Answer from the drawing. Dimensions are ordinates in mm from the lowest x, y and z of the part. A direction names the side the tool comes from. Give positions to 0.01 mm unless a question says otherwise; leave off trailing zeros. Write each loop counter-clockwise with the first axis right and the second up, starting at its lowest first coordinate (ties: lowest second). Pieces come first, ordered by that corner, then holes. Notation, with made-up numbers: M -1.5,18 L 20.5,18 A8 ccw 20.5,28 Z; hole C 9,4 d8. An arc over 180 degrees is marked long. Write each question's results on one line, items separated by ' | '. Start each with the question number.
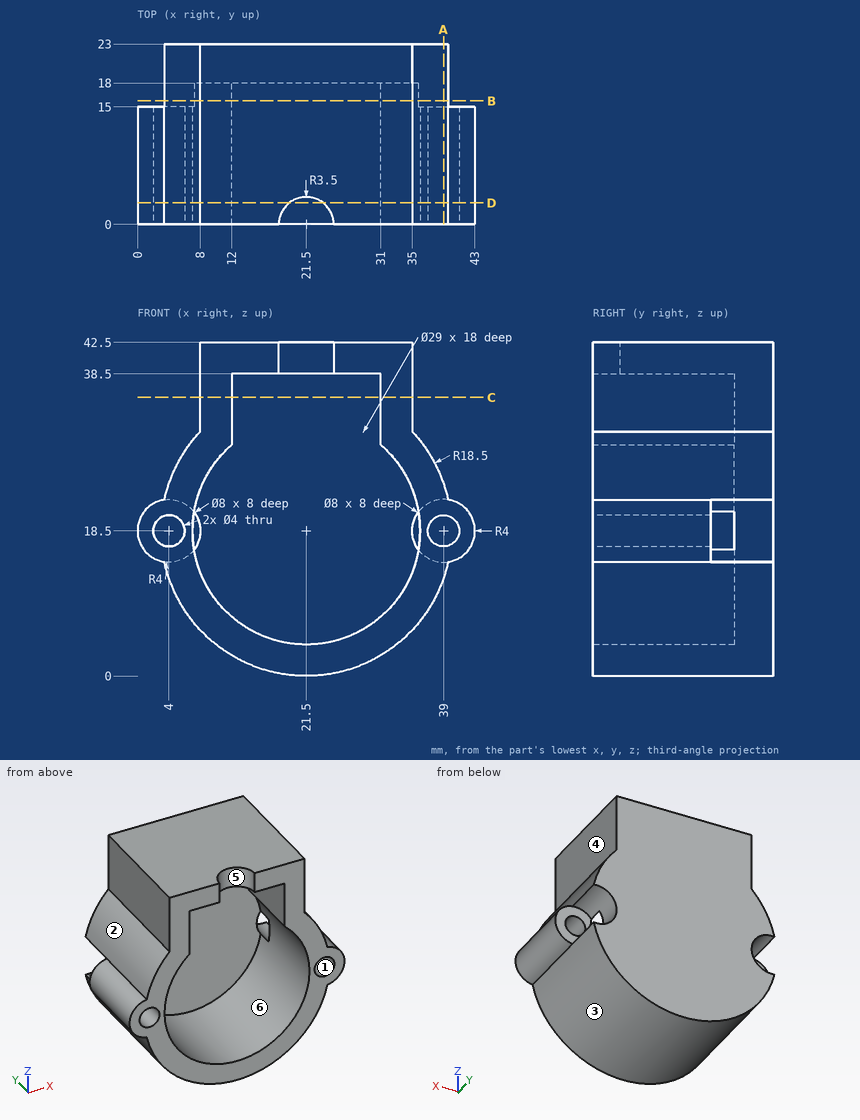
Item 1: Straight lines are drawn through the part: line 1 (X direction, y = 7.25, z = 18); line 2 (X direction, y = 16.25, z = 33); line 3 (Y direction, x = 27.5, z = 27.5). For each, find the intervals that lie inside material, in ascending order.
Item 2: For the marked faces 4, 5 and 6, determine the directions among +Z, -Z, +X, -X, +Y, -Y from which every point of the face is accessible in a straight line to the end or side of a thin tool.
Item 3: Section B-B, the plane y = 15.75 is taken. Determine the outline of the cut face in (x, z), then the cut area to 3 significant figures.
Item 4: Given P1, Ø3.5, axis at x = 3.5, z = 18.5, coming from the +Y side; P2, Ø5.5, axis at y = 9, z = 37.5, coming from the -X side; P3, Ø1.5, axis at y = 3, z = 27.5, coming from the +X side; P4, Ø3.5, axis at x = 4, z = 18.5, coming from the +Y side, each flat-ended and moving along its own axis, determine where each tip first touches the part or whether it passes through.
Item 5: Section C-C, the plane z = 35.5 is taken. Determine the outline of the cut face in (x, y).
Item 6: Determine the mould class of the marked faces 1, 2 and 3 for opening direction Z: +Z half, -Z half, draft (parallel to the pull), parting line (faces both ways), or undercut.
Item 7: Section A-A, the plane x = 39 is taken. Determine the outline of the cut face in (y, z).
Item 8: Section D-D, the plane y = 2.75 is taken. Determine the outline of the cut face in (x, z) (1 decimal).
Worked out:
1) line 1: x = 0.03 to 2.06, 5.94 to 7.01, 35.99 to 37.06, 40.94 to 42.97 | line 2: x = 8 to 12, 31 to 35 | line 3: y = 18 to 23
2) face 4: +Z, +X, +Y, -Y | face 5: +Z, -Y | face 6: -Y
3) outline: M 3.43,14.54 A18.5 ccw 39.57,14.54 A4 cw 35.8,16.1 A14.5 cw 7.2,16.1 A4 cw Z; M 3.43,22.46 A4 cw 7.2,20.9 A14.5 cw 12,29.45 L 12,38.5 L 31,38.5 L 31,29.45 A14.5 cw 35.8,20.9 A4 cw 39.57,22.46 A18.5 ccw 35,31.15 L 35,42.5 L 8,42.5 L 8,31.15 A18.5 ccw Z | area: 429 mm²
4) P1: stops at y = 15 | P2: stops at x = 8 | P3: stops at x = 38.06 | P4: passes through
5) outline: M 8,0 L 12,0 L 12,18 L 31,18 L 31,0 L 35,0 L 35,23 L 8,23 Z
6) face 1: undercut | face 2: +Z half | face 3: -Z half
7) outline: M 0,12.5 L 23,12.5 L 23,14.5 L 15,14.5 L 15,16.5 L 0,16.5 Z; M 0,20.5 L 15,20.5 L 15,22.5 L 23,22.5 L 23,24.5 L 0,24.5 Z
8) outline: M 3.4,14.5 A18.5 ccw 39.6,14.5 A4 ccw 39.6,22.5 A18.5 ccw 35,31.1 L 35,42.5 L 23.7,42.5 L 23.7,38.5 L 31,38.5 L 31,29.5 A14.5 cw long 12,29.5 L 12,38.5 L 19.3,38.5 L 19.3,42.5 L 8,42.5 L 8,31.1 A18.5 ccw 3.4,22.5 A4 ccw Z; hole C 4,18.5 d4; hole C 39,18.5 d4
